Autodesk Inventor part; units mm, degrees
ref_plane "YZ Plane" through (0, 0, 0) normal (1, 0, 0) x (0, 1, 0)
ref_plane "XZ Plane" through (0, 0, 0) normal (0, 1, 0) x (-1, 0, 0)
ref_plane "XY Plane" through (0, 0, 0) normal (0, 0, 1) x (1, 0, 0)
sketch "Эскиз1" plane through (0, 0, 0) normal (0, 0, 1) x (1, 0, 0)
  line L0 (-27, 0) -> (27, 0)
  line L1 (27, 0) -> (27, -5)
  line L2 (27, -5) -> (-27, -5)
  line L3 (-27, -5) -> (-27, 0)
  line L4 (27, -5) -> (22, -5)
  line L5 (22, -5) -> (22, -35)
  line L6 (22, -35) -> (27, -35)
  line L7 (27, -35) -> (27, -5)
  line L8 (-27, -5) -> (-22, -5)
  line L9 (-22, -5) -> (-22, -35)
  line L10 (-22, -35) -> (-27, -35)
  line L11 (-27, -35) -> (-27, -5)
  point P0 (0, 0)
  point P1 (0, 0)
  point P2 (-22, -5)
  point P3 (22, -5)
  dimension "d0" = 35
  dimension "d1" = 5
  dimension "d2" = 54
  dimension "d3" = 5
extrude "Выдавливание1" add sketch "Эскиз1" along normal blind 5
sketch "Эскиз3" plane through (-27, 0, 0) normal (0, 1, 0) x (1, 0, 0)
  line L0 (0, 0) -> (7, 0)
  line L1 (7, 0) -> (7, 20)
  line L2 (7, 20) -> (0, 20)
  line L3 (0, 20) -> (0, 0)
  line L4 (0, 20) -> (54, 20)
  line L5 (54, 20) -> (54, 27)
  line L6 (54, 27) -> (0, 27)
  line L7 (0, 27) -> (0, 20)
  line L8 (54, 0) -> (0, 0)
  line L9 (54, 20) -> (47, 20)
  line L10 (47, 20) -> (47, 0)
  line L11 (47, 0) -> (54, 0)
  line L12 (54, 0) -> (54, 20)
  line L13 (54, 0) -> (54, -5)
  point P0 (27, 0)
  point P1 (54, 0)
  dimension "d6" = 7
  dimension "d7" = 7
  dimension "d8" = 7
  dimension "d9" = 20
extrude "Выдавливание2" add sketch "Эскиз3" against normal blind 5 contours L3 L2 L1 L0 | L7 L6 L5 L4 L2 | L10 L4 L12 L8
sketch "Эскиз4" plane through (-27, 0, 5) normal (0, 1, 0) x (1, 0, 0)
  arc A0 (52.8363, 21.448) -> (52.8363, 18.648) centre (51.075, 20.048) ccw
  arc A1 (52.8363, 11.542) -> (52.8363, 8.742) centre (51.075, 10.142) ccw
  arc A2 (1.1636, 8.742) -> (1.1636, 11.542) centre (2.925, 10.142) ccw
  arc A3 (1.1636, 18.648) -> (1.1636, 21.448) centre (2.925, 20.048) ccw
  circle A4 centre (51.075, 20.048) radius 2.25
  circle A5 centre (51.075, 10.142) radius 2.25
  circle A6 centre (2.925, 10.142) radius 2.25
  circle A7 centre (2.925, 20.048) radius 2.25
  point P0 (27, 5)
  point P1 (1.1636, 21.448)
  point P2 (1.1636, 11.542)
  point P3 (52.8363, 8.742)
  point P4 (52.8363, 21.448)
extrude "Выдавливание3" cut sketch "Эскиз4" against normal blind 5
properties part number "держатель_сервы"
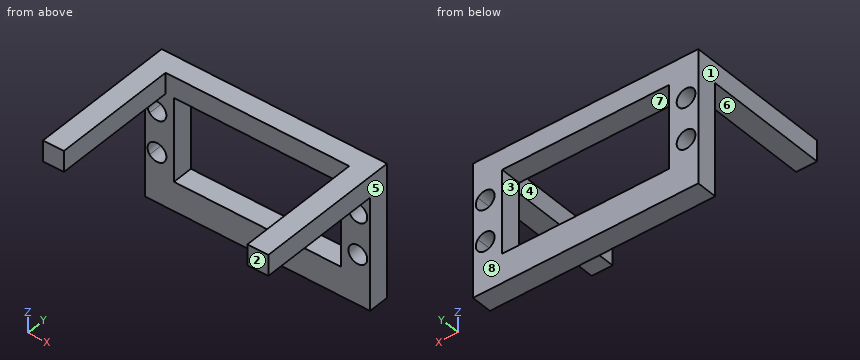
Source: CAD feature listing. Evaluate the final solid. Frame: model axes, mm. Face numbers are marked on the shaded views. A direction names the side the tool comes from. Coordinates: 2 decimals unless noted, no trailing zeros. Order: outer loops, then holes, each group sorted by start corner. A loop starts at its lowest first (then second) coordinate and runs counter-clockwise, first axis right, second up. Notation, with made-up numbers: M 74.25,58.5 L 109.25,58.5 A22 ccw 109.25,88.5 Z; hole C 32.5,64 d8. An arc over 180 degrees is marked long. Write each question's results on one line, items separated by ' | '. Start each with the question number.
Item 1: First-contact query: pin 1 Ø5.5 at (x, y) = (-24, -27) entering from -Z. Flat tip, straight axial feed; report the tip coordinate or a pass-through.
Item 2: Line query: probe 1 along Y at (x, z) = (-20.5, -5.5); probe 2 along X at (y, z) = (-3.5, -9); probe 3 along X at (y, z) = (-16.5, 0.5). Output: solid intervals per line, ascending.
Item 3: Cut plane D-D (z = -24). Return loops of the section in (x, y), and give its area (3 significant figures).
Item 4: Draft query along X for the marked faces 1, 2 and 3. Return one class per face: pulls with the +X half, pulls with the -X half, needs draft (parallel to the pull), parting line crosses it, or undercut.
Item 5: Cut plane C-C (z = 3). Return loops of the section in (x, y), and give its area (3 significant figures).
Item 6: Cut plane A-A (x = -9). Return loops of the section in (y, z).
Item 7: Set-up query: the marked faces 4, 5, 6, 7 and 8. Return all of +Z, -Z, +X, -X, +Y, -Y with unobstructed straight access to the full face (end or side cutting, diameter ignored); none if empty.
Item 8: Cut plane B-B (y = -23). Return loops of the section in (x, z), and give its area (3 significant figures).
Checked values:
1) pin 1: stops at z = 0
2) probe 1: y = -5 to 0 | probe 2: x = -27 to -20, 20 to 27 | probe 3: x = -27 to -22, 22 to 27
3) outline: M -27,-5 L 27,-5 L 27,0 L -27,0 Z | area: 270 mm2
4) face 1: pulls with the -X half | face 2: needs draft | face 3: undercut
5) outline: M -27,-35 L -22,-35 L -22,-5 L 22,-5 L 22,-35 L 27,-35 L 27,0 L -27,0 Z | area: 570 mm2
6) outline: M -5,-27 L 0,-27 L 0,-20 L -5,-20 Z; M -5,0 L 0,0 L 0,5 L -5,5 Z
7) face 4: +Z, -Z, -Y | face 5: +Z, -Z, +X, +Y, -Y | face 6: -Z, +X, -X, -Y | face 7: +Y, -Y | face 8: +Z, -Z, +X, -X, +Y
8) outline: M -27,0 L -22,0 L -22,5 L -27,5 Z; M 22,0 L 27,0 L 27,5 L 22,5 Z | area: 50.0 mm2
